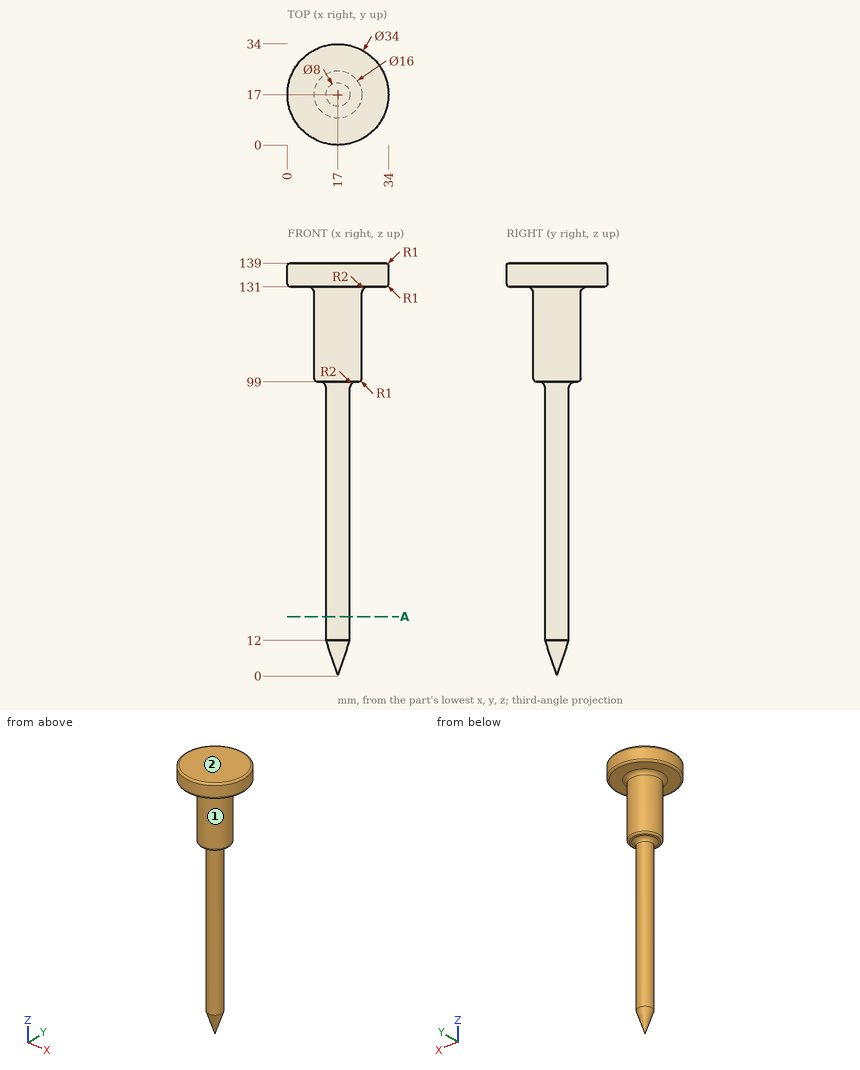
Geometry check sheet. Reference: drawing and pictorial views, mm from the part's lowest x, y, z. A direction names the side the tool comes from. Give positions to 0.01 mm unless a question says otherwise; leave off trailing zeros. Loops run counter-clockwise (first coordinate to the right, second up) from the corner with the lowest first, then second, coordinate; pieces in that order, holes last. Notation, with made-up numbers: (-35.75, 68.5) -> (8.25, 68.5) arc R15 ccw to (8.25, 96.5) -> close; hole circle Ø4 at (42, 71). An arc over 180 degrees is marked (long way). Answer in a Markdown table with one row per item. Add a question column.
1) Gauge pin test, flat ends, axial feed: P1, Ø3, axis at x = 9.5, y = 24, coming from the -Z side; P2, Ø6, axis at y = 9, z = 106, coming from the -X side (3 decimals); P3, Ø8, axis at x = 19.5, z = 38, coming from the -Y side. Record the tip position at first contact, or that the pin passes through.
2) Set-up check for the marked faces 1 and 2: record each of +Z, -Z, +X, -X, +Y, -Y from which the full face is reachable in a straight line by a thin tool's end or side.
3) Material ranges on probe 1 along Z at (x, y) = (5.5, 10); probe 2 along Z at (x, y) = (11.5, 19.5); probe 3 along Y at (x, z) = (17.5, 34.5), recorded low to high. Write a range as from..to.
4) Cross-section at A-A on z = 20. Record the boundary of the cut face in (x, y), and give its area (3 significant figures).
Outcome:
| question | item | result |
|---|---|---|
| 1 | P1 | stops at z = 130.57 |
| 1 | P2 | stops at x = 10.755 |
| 1 | P3 | stops at y = 13 |
| 2 | face 1 | -Z |
| 2 | face 2 | +Z, +X, -X, +Y, -Y |
| 3 | probe 1 | z = 131..139 |
| 3 | probe 2 | z = 99..139 |
| 3 | probe 3 | y = 13.03..20.97 |
| 4 | outline | circle Ø8 at (17, 17) |
| 4 | area | 50.3 mm^2 |
